Geometry check sheet. Reference: the model listing, model coordinates, mm. A direction names the side the tool comes from. Give positions to 0.01 mm unless a question says otherwise; leave off trailing zeros. Write each loop counter-clockwise with the first axis right and the second up, starting at its lowest first coordinate (ties: lowest second). Pieces come first, ordered by that corner, then holes. Notation, with made-up numbers: (78.25, 0.5) - (113.25, 0.5) arc R28 cw to (113.25, 39.5) - close; hole circle Ø8 at (21, 27.25). An arc over 180 degrees is marked (long way). One line per question, with ' | ' between items. Start each with the question number.
Q1. Set-up check for faces 4 (the face through (-35, -16, 2)), 5 (the face through (41.71, 51.48, 1.97)), 6 (the face through (30.74, -3.65, 1.23)), 7 (the face through (150, -13, 2)), 8 (the face through (-18, -13.5, 2)): record each of +Z, -Z, +X, -X, +Y, -Y from which the full face is reachable in a straight line by a thin tool's end or side.
Q2. Release check for a two-part mould opening along X. For faces 1 (the face through (-29, 13.5, 2)), 2 (the face through (13.497, -0.297, 1.972)), 3 (the face through (53.12, 72.11, 1.97)) record: +X half, -X half, draft (parallel to the pull), parting line (faces both ways), or undercut.
Q3. Section check A-A on y = 0. Record the boundary of the cut face in (x, z), and give its area (3 significant figures).
Q4. Section check D-D on x = 104. Record the boundary of the cut face in (y, z), and give its area (3 significant figures).
Q5. Gauge pin test, flat ends, axial feed: P1, Ø1, axis at y = 68.5, z = 2.5, coming from the +X side; P2, Ø1.5, axis at x = 9, z = 3, coming from the +Y side. Record the tip position at first contact, or that the pin passes through.
Q6. Section check C-C on z = 1.6. Record the boundary of the cut face in (x, y).
Q7. Section check B-B on x = 55.5. Record the boundary of the cut face in (y, z), and give its area (3 significant figures).
Q8. Thickness scan on L1, parallel to Y at x = 54, z = 0.75; L2, parallel to Y at x = 35.5, z = 0.6; L3, parallel to Y at x = 65, z = 1.8. Record the ranges inside material, lowest first. Write a range as [from, to].
```python
from build123d import *

# Parameters (mm, degrees)
SKETCH_1_R             = 3
SKETCH_1_R_2           = 6
SM_BASE_FLANGE_1_DEPTH = 4
CHAMFER_2_SIZE         = 1.5


# Sheet-metal steps are written as plain solids
with BuildPart() as part:
    # Sketch 1 → Базовая кромка1 (new body)
    with BuildSketch(Plane.XY):
        with BuildLine():
            Line((60.509861789, 68.353533944), (22.375898858, 34.12410114))
            Line((22.375898858, 34.12410114), (47.171572875, 6.5))
            Line((47.171572875, 6.5), (150, 6.5))
            Line((150, 6.5), (150, -33.5))
            Line((150, -33.5), (14.5, -33.5))
            Line((14.5, -33.5), (-35, -18.5))
            Line((-35, -18.5), (-35, -13.5))
            Line((-35, -13.5), (0, -13.5))
            ThreePointArc((0, -13.5), (13.5, 0), (0, 13.5))
            Line((0, 13.5), (-58.308631084, 13.5))
            Line((-58.308631084, 13.5), (-75.090623708, 33.5))
            Line((-75.090623708, 33.5), (52.891961096, 80.966804205))
            ThreePointArc((52.891961096, 80.966804205), (61.919955994, 77.812259079), (60.509861789, 68.353533944))
        make_face()
        with Locations((55.5, 73.934867553)):
            Circle(SKETCH_1_R, mode=Mode.SUBTRACT)
        with Locations((35.5, 0)):
            Circle(SKETCH_1_R_2, mode=Mode.SUBTRACT)
    extrude(amount=SM_BASE_FLANGE_1_DEPTH)

    # Фаска2
    chamfer_2_edges = [part.edges().sort_by_distance(p)[0] for p in [
        (29.5, 0, 4),
    ]]
    chamfer(chamfer_2_edges, length=CHAMFER_2_SIZE)


solid = part.part
```
Working result:
1) face 4: +Z, -Z, -X, -Y | face 5: +Z, -Z, +X | face 6: +Z, -Z | face 7: +Z, -Z, +X, +Y, -Y | face 8: +Z, -Z, -X
2) face 1: draft | face 2: -X half | face 3: undercut
3) outline: (13.5, 0) - (29.5, 0) - (29.5, 2.5) - (28, 4) - (13.5, 4) - close; (41.5, 0) - (150, 0) - (150, 4) - (43, 4) - (41.5, 2.5) - close | area: 496 mm2
4) outline: (-33.5, 0) - (6.5, 0) - (6.5, 4) - (-33.5, 4) - close | area: 160 mm2
5) P1: stops at x = 61.15 | P2: stops at y = 64.97
6) outline: (-75.09, 33.5) - (-58.31, 13.5) - (0, 13.5) arc R13.5 cw to (0, -13.5) - (-35, -13.5) - (-35, -18.5) - (14.5, -33.5) - (150, -33.5) - (150, 6.5) - (47.17, 6.5) - (22.38, 34.12) - (60.51, 68.35) arc R7.5 ccw to (52.89, 80.97) - close; hole circle Ø12 at (35.5, 0); hole circle Ø6 at (55.5, 73.93)
7) outline: (-33.5, 0) - (6.5, 0) - (6.5, 4) - (-33.5, 4) - close; (63.86, 0) - (70.93, 0) - (70.93, 4) - (63.86, 4) - close; (76.93, 0) - (81.43, 0) - (81.43, 4) - (76.93, 4) - close | area: 206 mm2
8) L1: y = [-33.5, 6.5], [62.51, 71.34], [76.53, 81.28] | L2: y = [-33.5, -6], [6, 19.5], [45.9, 74.52] | L3: y = [-33.5, 6.5]
